Geometry check sheet. Reference: the model listing, model coordinates, mm. Face numbers are marked on the shaded views. A direction names the side the tool comes from. Coordinates: 2 decimals unless noted, no trailing zeros. Loops run counter-clockwise (first coordinate to the right, second up) from the corner with the lowest first, then second, coordinate; pieces in that order, holes last.
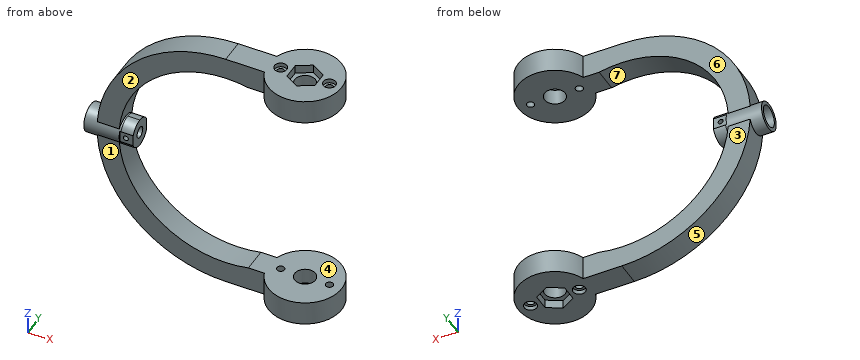
from build123d import *

# Parameters (mm, degrees)
BOSS_EXTRUDE1_DEPTH      = 10
BOSS_EXTRUDE1_DEPTH_BACK = 10
SKETCH2_R                = 30
BOSS_EXTRUDE2_DEPTH      = 20
CUT_EXTRUDE1_REACH       = 239.805
SKETCH3_R                = 8.5
SKETCH3_R_2              = 3.05
CUT_EXTRUDE3_DEPTH       = 155.468443379
SKETCH7_R                = 8.5
CUT_EXTRUDE4_DEPTH       = 7
SKETCH8_R                = 11.75
BOSS_EXTRUDE3_DEPTH      = 10
BOSS_EXTRUDE3_DEPTH_BACK = 20
SKETCH9_R                = 8.75
CUT_EXTRUDE5_DEPTH       = 8
SKETCH10_R               = 4.57
CUT_EXTRUDE6_DEPTH       = 226.912593764
SKETCH11_R               = 11.75
SKETCH11_R_2             = 4.57
BOSS_EXTRUDE4_DEPTH      = 10
SKETCH12_R               = 2.05
CUT_EXTRUDE7_DEPTH       = 160.281198025
CUT_EXTRUDE7_DEPTH_BACK  = 160.281198025
SKETCH13_R               = 5.1
SKETCH13_R_2             = 3.05
CUT_EXTRUDE8_DEPTH       = 3.5
SKETCH14_W               = 11
SKETCH14_H               = 23.5
CUT_EXTRUDE9_DEPTH       = 1


with BuildPart() as part:
    # Sketch1 → Boss-Extrude1 (new, two sides)
    with BuildSketch(Plane(origin=(0, 0, 0), x_dir=(1, 0, 0), z_dir=(0, 1, 0))) as boss_extrude1_sk:
        with BuildLine():
            Line((80, 105.5), (0, 105.5))
            ThreePointArc((0, 105.5), (-105.5, 0), (0, -105.5))
            Line((0, -105.5), (80, -105.5))
            Line((80, -105.5), (80, -85.5))
            Line((80, -85.5), (0, -85.5))
            ThreePointArc((0, -85.5), (-85.5, 0), (0, 85.5))
            Line((0, 85.5), (80, 85.5))
            Line((80, 85.5), (80, 105.5))
        make_face()
    extrude(amount=BOSS_EXTRUDE1_DEPTH)
    extrude(boss_extrude1_sk.sketch, amount=-BOSS_EXTRUDE1_DEPTH_BACK)

    # Sketch2 → Boss-Extrude2 (add)
    with BuildSketch(Plane.XY.offset(105.5)):
        with Locations((60, 0)):
            Circle(SKETCH2_R)
    boss_extrude2 = extrude(amount=-BOSS_EXTRUDE2_DEPTH)

    # Sketch3 → Cut-Extrude1 (cut, up to next)
    with BuildSketch(Plane.XY.offset(105.5), mode=Mode.PRIVATE) as cut_extrude1_sk1:
        with Locations((60, 0)):
            Circle(SKETCH3_R)
    cut_extrude1_tool1 = extrude(cut_extrude1_sk1.sketch, amount=-CUT_EXTRUDE1_REACH, mode=Mode.PRIVATE) & part.part
    # Sketch3 → Cut-Extrude1 (cut, up to next)
    with BuildSketch(Plane.XY.offset(105.5), mode=Mode.PRIVATE) as cut_extrude1_sk2:
        with Locations((80, 0)):
            Circle(SKETCH3_R_2)
    cut_extrude1_tool2 = extrude(cut_extrude1_sk2.sketch, amount=-CUT_EXTRUDE1_REACH, mode=Mode.PRIVATE) & part.part
    # Sketch3 → Cut-Extrude1 (cut, up to next)
    with BuildSketch(Plane.XY.offset(105.5), mode=Mode.PRIVATE) as cut_extrude1_sk3:
        with Locations((40, 0)):
            Circle(SKETCH3_R_2)
    cut_extrude1_tool3 = extrude(cut_extrude1_sk3.sketch, amount=-CUT_EXTRUDE1_REACH, mode=Mode.PRIVATE) & part.part
    cut_extrude1_1 = cut_extrude1_tool1.solids().sort_by_distance((60, 0, 105.5))[0]
    add(cut_extrude1_1, mode=Mode.SUBTRACT)
    cut_extrude1_2 = cut_extrude1_tool2.solids().sort_by_distance((80, 0, 105.5))[0]
    add(cut_extrude1_2, mode=Mode.SUBTRACT)
    cut_extrude1_3 = cut_extrude1_tool3.solids().sort_by_distance((40, 0, 105.5))[0]
    add(cut_extrude1_3, mode=Mode.SUBTRACT)
    cut_extrude1 = cut_extrude1_1 + cut_extrude1_2 + cut_extrude1_3  # Cut-Extrude1 as one shape, for the pattern or mirror that repeats it

    # Mirror2: Boss-Extrude2, Cut-Extrude1 across plane
    add(boss_extrude2.mirror(Plane.XY))
    add(cut_extrude1.mirror(Plane.XY), mode=Mode.SUBTRACT)

    # Sketch6 → Cut-Extrude3 (cut, through all)
    with BuildSketch(Plane(origin=(0, 10, 0), x_dir=(1, 0, 0), z_dir=(0, 1, 0))):
        with BuildLine():
            Line((31.715728753, 81.549755056), (31.715728753, -81.549755056))
            ThreePointArc((31.715728753, -81.549755056), (-87.5, 0), (31.715728753, 81.549755056))
        make_face()
    extrude(amount=-CUT_EXTRUDE3_DEPTH, mode=Mode.SUBTRACT)

    # Sketch7 → Cut-Extrude4 (cut)
    with BuildSketch(Plane.XY.offset(105.5)):
        Polygon((60, 13.279056191), (48.5, 6.639528096), (48.5, -6.639528096), (60, -13.279056191), (71.5, -6.639528096), (71.5, 6.639528096), align=None)
        with Locations((60, 0)):
            Circle(SKETCH7_R, mode=Mode.SUBTRACT)
    cut_extrude4 = extrude(amount=-CUT_EXTRUDE4_DEPTH, mode=Mode.SUBTRACT)

    # Mirror3: Cut-Extrude4 across plane
    add(cut_extrude4.mirror(Plane.XY), mode=Mode.SUBTRACT)

    # Sketch8 → Boss-Extrude3 (add, two sides)
    with BuildSketch(Plane.ZY.offset(105.5)) as boss_extrude3_sk:
        Circle(SKETCH8_R)
    extrude(amount=BOSS_EXTRUDE3_DEPTH)
    extrude(boss_extrude3_sk.sketch, amount=-BOSS_EXTRUDE3_DEPTH_BACK)

    # Sketch9 → Cut-Extrude5 (cut)
    with BuildSketch(Plane.ZY.offset(115.5)):
        Circle(SKETCH9_R)
    extrude(amount=-CUT_EXTRUDE5_DEPTH, mode=Mode.SUBTRACT)

    # Sketch10 → Cut-Extrude6 (cut, through all)
    with BuildSketch(Plane.ZY.offset(107.5)):
        Circle(SKETCH10_R)
    extrude(amount=-CUT_EXTRUDE6_DEPTH, mode=Mode.SUBTRACT)

    # Sketch11 → Boss-Extrude4 (add)
    with BuildSketch(Plane(origin=(-85.5, 0, 0), x_dir=(0, 0, -1), z_dir=(1, 0, 0))):
        with Locations(Location((0, 0, 0), (0, 0, 180))):
            Circle(SKETCH11_R)
        with Locations(Location((0, 0, 0), (0, 0, 180))):
            Circle(SKETCH11_R_2, mode=Mode.SUBTRACT)
    extrude(amount=BOSS_EXTRUDE4_DEPTH)

    # Sketch12 → Cut-Extrude7 (cut, two sides)
    with BuildSketch(Plane(origin=(0, 0, 0), x_dir=(1, 0, 0), z_dir=(0, 1, 0))) as cut_extrude7_sk:
        with Locations(Location((-81.5, 0, 0), (0, 0, 270))):
            Circle(SKETCH12_R)
    extrude(amount=CUT_EXTRUDE7_DEPTH, mode=Mode.SUBTRACT)
    extrude(cut_extrude7_sk.sketch, amount=-CUT_EXTRUDE7_DEPTH_BACK, mode=Mode.SUBTRACT)

    # Sketch13 → Cut-Extrude8 (cut)
    with BuildSketch(Plane.XY.offset(105.5)):
        with Locations((40, 0)):
            Circle(SKETCH13_R)
        with Locations((40, 0)):
            Circle(SKETCH13_R_2, mode=Mode.SUBTRACT)
        with Locations((80, 0)):
            Circle(SKETCH13_R)
        with Locations((80, 0)):
            Circle(SKETCH13_R_2, mode=Mode.SUBTRACT)
    cut_extrude8 = extrude(amount=-CUT_EXTRUDE8_DEPTH, mode=Mode.SUBTRACT)

    # Mirror4: Cut-Extrude8 across plane
    add(cut_extrude8.mirror(Plane.XY), mode=Mode.SUBTRACT)

    # Sketch14 → Cut-Extrude9 (cut)
    with BuildSketch(Plane(origin=(0, 11.75, 0), x_dir=(1, 0, 0), z_dir=(0, 1, 0))):
        with Locations((-81, 0)):
            Rectangle(SKETCH14_W, SKETCH14_H)
    cut_extrude9 = extrude(amount=-CUT_EXTRUDE9_DEPTH, mode=Mode.SUBTRACT)

    # Mirror5: Cut-Extrude9 across plane
    add(cut_extrude9.mirror(Plane.ZX), mode=Mode.SUBTRACT)


solid = part.part
1) Section check C-C on x = 40. Record the cut outline in (y, z), and give its area (3 significant figures).
Data:
outline: (-22.36, -105.5) - (-5.1, -105.5) - (-5.1, -102) - (-3.05, -102) - (-3.05, -85.5) - (-22.36, -85.5) - close; (-22.36, 85.5) - (-3.05, 85.5) - (-3.05, 102) - (-5.1, 102) - (-5.1, 105.5) - (-22.36, 105.5) - close; (3.05, -102) - (5.1, -102) - (5.1, -105.5) - (22.36, -105.5) - (22.36, -85.5) - (3.05, -85.5) - close; (3.05, 85.5) - (22.36, 85.5) - (22.36, 105.5) - (5.1, 105.5) - (5.1, 102) - (3.05, 102) - close
area: 1,520 mm2
2) Material ranges on probe 1 along Y at (x, z) = (-113, 0); probe 2 along Z at (x, y) = (-81, 8); probe 3 along Y at (x, z) = (60, -94.75), recorded low to high.
Data:
probe 1: y = -11.75 to -8.75, 8.75 to 11.75
probe 2: z = -67.6 to -33.09, -8.61 to -1.99, 1.99 to 8.61, 33.09 to 67.6
probe 3: y = -30 to -8.5, 8.5 to 30
3) Depth check by flat-ended pin: pin 1 (10 mm diameter, centred on x = 80, y = 0, fed in from +Z); pin 2 (3 mm diameter, centred on x = 79.5, y = -1, fed in from +Z); pin 3 (4.5 mm diameter, centred on x = -81.5, z = 0.5, fed in from +Y); pin 4 (4 mm diameter, centred on x = -71, y = 5.5, fed in from -Z). Enter the tip coordinate at first touch or a pass-through.
Data:
pin 1: stops at z = 102
pin 2: passes through
pin 3: stops at y = 10.75
pin 4: stops at z = -79.81
4) Section check D-D on x = -91. Record the cut outline in (y, z).
Data:
outline: (-10, -53.38) - (10, -53.38) - (10, -6.17) arc R11.75 ccw to (10, 6.17) - (10, 53.38) - (-10, 53.38) - (-10, 6.17) arc R11.75 ccw to (-10, -6.17) - close; hole circle Ø9.14 at (0, 0)
5) Access from +Z, -Z, +X, -X, +Y, -Y to the whole of each face (thin tool, end or side, straight path). Record for the marked faces 1, 2, 3 and 4.
Data:
face 1: -Z, -X, -Y
face 2: +Z, -X, -Y
face 3: -Z, -X, +Y
face 4: +X, +Y, -Y
6) Section check A-A on x = 15.5. Record the cut outline in (y, z), and give its area (3 significant figures).
Data:
outline: (-10, -105.5) - (10, -105.5) - (10, -86.12) - (-10, -86.12) - close; (-10, 86.12) - (10, 86.12) - (10, 105.5) - (-10, 105.5) - close
area: 775 mm2
7) Section check B-B on y = -17. Record the cut outline in (x, z), and give its area (3 significant figures).
Data:
outline: (35.28, -105.5) - (84.72, -105.5) - (84.72, -85.5) - (35.28, -85.5) - close; (35.28, 85.5) - (84.72, 85.5) - (84.72, 105.5) - (35.28, 105.5) - close
area: 1,980 mm2
8) Mould release check, pull along Z, two halves, no side actions. Record for the marked faces 5, 6 and 7: +Z half, -Z half, draft (parallel to the pull), parting line (faces both ways), or undercut.
Data:
face 5: -Z half
face 6: draft
face 7: undercut
